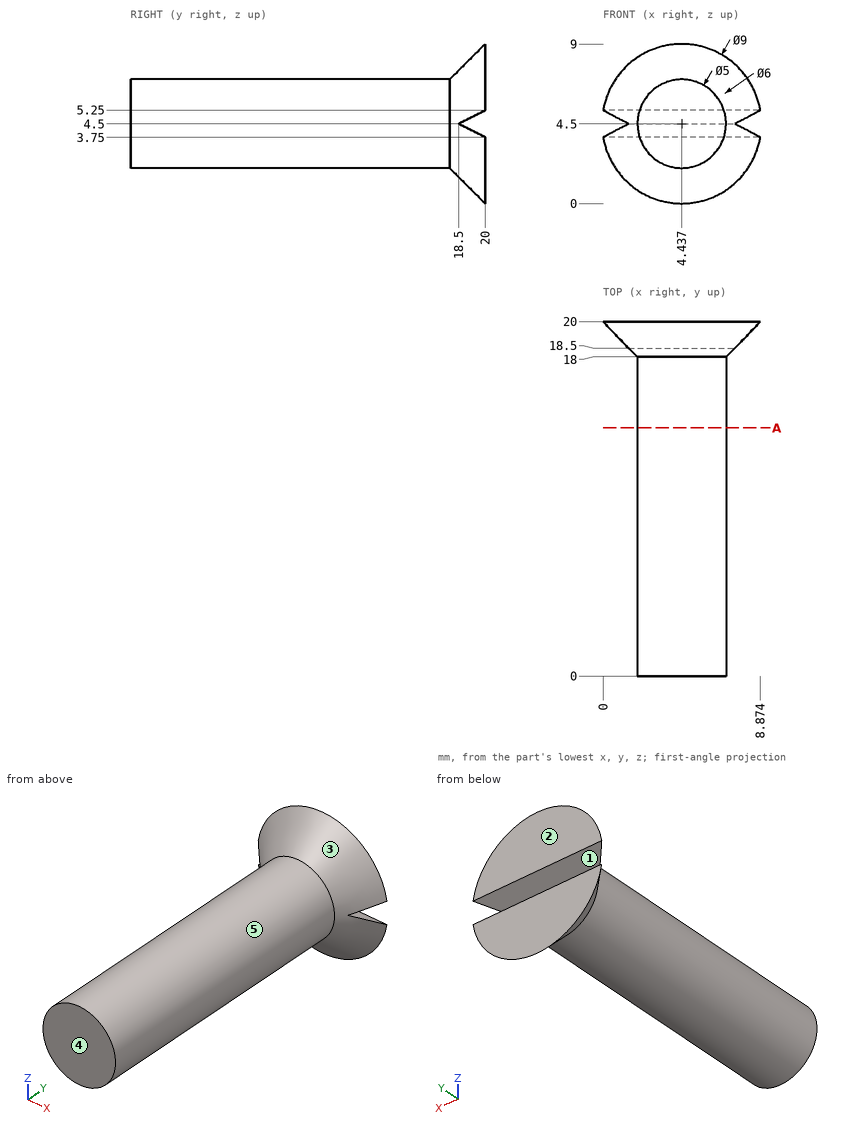
Design review of the part shown in the three views and the two pictorial views. Dimensions are in mm from the part's minimum x, y and z. A direction names the side the tool comes from. Round coordinates to 2 decimals unless told otherwise and drop trailing zeros. Loops run counter-clockwise (first coordinate to the right, second up) from the corner with the lowest first, then second, coordinate; pieces in that order, holes last.
1) Consider section A-A on y = 14. State the section outline as (x, z) points.
Values follow:
outline: circle Ø5 at (4.44, 4.5)
2) Tool access review of the marked faces 4 and 5: name each direction out of +Z, -Z, +X, -X, +Y, -Y from which nothing blocks a thin tool from reaching the whole face with its end or side.
Values follow:
face 4: +Z, -Z, +X, -X, -Y
face 5: -Y
3) The part is to be moulded in two halves that separate along Z. For the marked faces 1, 2 and 3, say which applies: pulls with the +Z half, pulls with the -Z half, needs draft (parallel to the pull), parting line crosses it, or undercut.
Values follow:
face 1: undercut
face 2: needs draft
face 3: parting line crosses it
4) Wall thickness on line 1 along Y through (x, z) = (3.5, 4); line 2 along Z through (x, y) = (3.25, 6.5); line 3 along Y through (x, z) = (6.5, 1.25): over which ranges is each line inside the solid? List them lowest first.
Values follow:
line 1: y = 0 to 19.5
line 2: z = 2.3 to 6.7
line 3: y = 19.35 to 20
5) Clearance check with flat-ended pins moving along their axes: P1, Ø3, axis at y = 2.5, z = 8, coming from the -X side; P2, Ø5, axis at x = 6.5, y = 7.5, coming from the -Z side; P3, Ø3, axis at x = 6.5, y = 8, coming from the +Z side. State where each tip first meets the part, or that it passes through.
Values follow:
P1: stops at x = 2.94
P2: stops at z = 2
P3: stops at z = 6.94
